Source: CAD feature listing. Evaluate the final solid. Frame: model axes, mm. Round coordinates to 2 decimals unless told otherwise and drop trailing zeros. Loops run counter-clockwise (first coordinate to the right, second up) from the corner with the lowest first, then second, coordinate; pieces in that order, holes last. Notation, with made-up numbers: (18, -24) - (34, -24) arc R15 cw to (34, -12) - close; hole circle Ø9 at (65.5, -11). An arc over 180 degrees is marked (long way). One line per question, with ' | ' between items. Start each with the question number.
1. Pin query (flat end, axial travel): pin 1 (3 mm diameter, centred on x = 110.5, y = 5, fed in from -Z); pin 2 (19.5 mm diameter, centred on x = -34, y = -6, fed in from +Z). Return the tip coordinate at first contact, or that it passes through.
2. Cut plane D-D (y = 47.5). Return loops of the section in (x, z), then the cut area to 3 significant figures.
3. Cut plane A-A (x = -30). Return loops of the section in (y, z).
4. Cut plane C-C (x = 28.5). Return loops of the section in (y, z).
5. Ray query, line 1 (X direction, y = 77, z = 1.25); line 2 (X direction, y = 3.5, z = 5.5); line 3 (Y direction, x = 62.5, z = 2.25). Return the intervals inside material, ascending.
6. Cut plane B-B (z = 3). State how many separate pieces and enclosed holes the cut face has, then the cut area to 3 significant figures.
```python
from build123d import *

# Parameters (mm, degrees)
F0_W     = 230
F0_H     = 140
F1_DEPTH = 12
F2_R     = 19.375
F2_R_2   = 10
F3_DEPTH = 7
F4_DEPTH = 25


with BuildPart() as f1:
    # F0 (on Top) → F1 (new body)
    with BuildSketch(Plane.XY):
        with Locations((57.0600198209, 31.2740390003)):
            Rectangle(F0_W, F0_H)
    extrude(amount=F1_DEPTH)

    # F2 (on face) → F3 (cut)
    with BuildSketch(Plane.XY.offset(12)):
        with Locations((-32.9399801791, 76.2740390003)):
            Circle(F2_R)
        with Locations((-32.9399801791, 76.2740390003)):
            Circle(F2_R_2, mode=Mode.SUBTRACT)
        with Locations((-32.9399801791, 31.2740390003)):
            Circle(F2_R)
        with Locations((-32.9399801791, 31.2740390003)):
            Circle(F2_R_2, mode=Mode.SUBTRACT)
        with Locations((-32.9399801791, -13.7259609997)):
            Circle(F2_R)
        with Locations((-32.9399801791, -13.7259609997)):
            Circle(F2_R_2, mode=Mode.SUBTRACT)
        with Locations((12.0600198209, -13.7259609997)):
            Circle(F2_R)
        with Locations((12.0600198209, -13.7259609997)):
            Circle(F2_R_2, mode=Mode.SUBTRACT)
        with Locations((12.0600198209, 31.2740390003)):
            Circle(F2_R)
        with Locations((12.0600198209, 31.2740390003)):
            Circle(F2_R_2, mode=Mode.SUBTRACT)
        with Locations((12.0600198209, 76.2740390003)):
            Circle(F2_R)
        with Locations((12.0600198209, 76.2740390003)):
            Circle(F2_R_2, mode=Mode.SUBTRACT)
        with Locations((57.0600198209, 76.2740390003)):
            Circle(F2_R)
        with Locations((57.0600198209, 76.2740390003)):
            Circle(F2_R_2, mode=Mode.SUBTRACT)
        with Locations((57.0600198209, 31.2740390003)):
            Circle(F2_R)
        with Locations((57.0600198209, 31.2740390003)):
            Circle(F2_R_2, mode=Mode.SUBTRACT)
        with Locations((57.0600198209, -13.7259609997)):
            Circle(F2_R)
        with Locations((57.0600198209, -13.7259609997)):
            Circle(F2_R_2, mode=Mode.SUBTRACT)
        with Locations((102.0600198209, -13.7259609997)):
            Circle(F2_R)
        with Locations((102.0600198209, -13.7259609997)):
            Circle(F2_R_2, mode=Mode.SUBTRACT)
        with Locations((102.0600198209, 31.2740390003)):
            Circle(F2_R)
        with Locations((102.0600198209, 31.2740390003)):
            Circle(F2_R_2, mode=Mode.SUBTRACT)
        with Locations((102.0600198209, 76.2740390003)):
            Circle(F2_R)
        with Locations((102.0600198209, 76.2740390003)):
            Circle(F2_R_2, mode=Mode.SUBTRACT)
        with Locations((147.0600198209, 76.2740390003)):
            Circle(F2_R)
        with Locations((147.0600198209, 76.2740390003)):
            Circle(F2_R_2, mode=Mode.SUBTRACT)
        with Locations((147.0600198209, 31.2740390003)):
            Circle(F2_R)
        with Locations((147.0600198209, 31.2740390003)):
            Circle(F2_R_2, mode=Mode.SUBTRACT)
        with Locations((147.0600198209, -13.7259609997)):
            Circle(F2_R)
        with Locations((147.0600198209, -13.7259609997)):
            Circle(F2_R_2, mode=Mode.SUBTRACT)
    extrude(amount=-F3_DEPTH, mode=Mode.SUBTRACT)

    # F4 (cut): faces of the model
    f4_faces = [f1.faces().sort_by_distance(p)[0] for p in [
        (-32.9399801791, 76.2740390003, 12),
        (12.0600198209, 76.2740390003, 12),
        (57.0600198209, 76.2740390003, 12),
        (102.0600198209, 76.2740390003, 12),
        (147.0600198209, 76.2740390003, 12),
        (147.0600198209, 31.2740390003, 12),
        (102.0600198209, 31.2740390003, 12),
        (57.0600198209, 31.2740390003, 12),
        (12.0600198209, 31.2740390003, 12),
        (-32.9399801791, 31.2740390003, 12),
        (-32.9399801791, -13.7259609997, 12),
        (12.0600198209, -13.7259609997, 12),
        (57.0600198209, -13.7259609997, 12),
        (102.0600198209, -13.7259609997, 12),
        (147.0600198209, -13.7259609997, 12),
    ]]
    extrude(f4_faces, amount=-F4_DEPTH, mode=Mode.SUBTRACT)


solid = f1.part
```
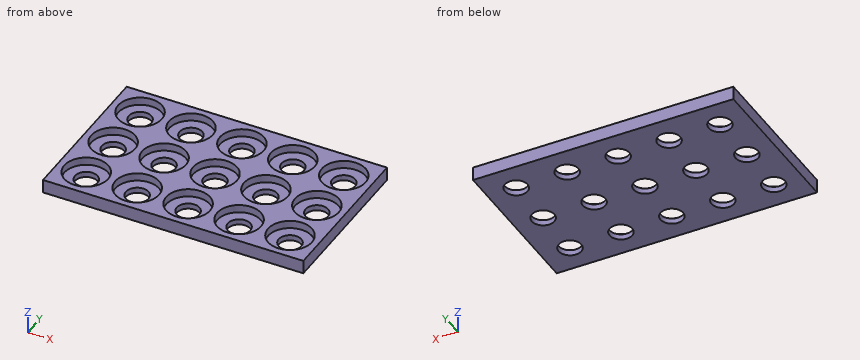
Answers follow:
1) pin 1: stops at z = 0 | pin 2: stops at z = 5
2) outline: (-57.94, 0) - (172.06, 0) - (172.06, 12) - (157.65, 12) - (157.65, 5) - (136.47, 5) - (136.47, 12) - (112.65, 12) - (112.65, 5) - (91.47, 5) - (91.47, 12) - (67.65, 12) - (67.65, 5) - (46.47, 5) - (46.47, 12) - (22.65, 12) - (22.65, 5) - (1.47, 5) - (1.47, 12) - (-22.35, 12) - (-22.35, 5) - (-43.53, 5) - (-43.53, 12) - (-57.94, 12) - close | area: 2,020 mm2
3) outline: (-38.73, 0) - (-23.28, 0) - (-23.28, 5) - (-32.88, 5) - (-32.88, 12) - (-38.73, 12) - close; (-4.17, 0) - (21.72, 0) - (21.72, 5) - (12.12, 5) - (12.12, 12) - (5.42, 12) - (5.42, 5) - (-4.17, 5) - close; (40.83, 0) - (66.72, 0) - (66.72, 5) - (57.12, 5) - (57.12, 12) - (50.42, 12) - (50.42, 5) - (40.83, 5) - close; (85.83, 0) - (101.27, 0) - (101.27, 12) - (95.42, 12) - (95.42, 5) - (85.83, 5) - close
4) outline: (-38.73, 0) - (101.27, 0) - (101.27, 12) - (86.53, 12) - (86.53, 5) - (66.02, 5) - (66.02, 12) - (41.53, 12) - (41.53, 5) - (21.02, 5) - (21.02, 12) - (-3.47, 12) - (-3.47, 5) - (-23.98, 5) - (-23.98, 12) - (-38.73, 12) - close
5) line 1: x = -57.94 to -42.91, -22.97 to 2.09, 22.03 to 47.09, 67.03 to 92.09, 112.03 to 137.09, 157.03 to 172.06 | line 2: x = -57.94 to -41.81, -24.07 to 3.19, 20.93 to 48.19, 65.93 to 93.19, 110.93 to 138.19, 155.93 to 172.06 | line 3: y = -38.73 to -22.12, -5.34 to 22.88, 39.66 to 67.88, 84.66 to 101.27
6) separate pieces: 1 | enclosed holes: 15 | area: 27,500 mm2
